```python
from build123d import *

# Parameters (mm, degrees)
F0_R     = 1.27
F1_DEPTH = 1.5875
F0_W     = 8.382
F0_H     = 7.62
F0_W_2   = 0.762
F2_DEPTH = 6.35
F0_W_3   = 11.811
F0_H_2   = 9.017
F0_W_4   = 3.048
F3_DEPTH = 9.525


with BuildPart() as f1:
    # F0 (on Top) → F1 (new body)
    with BuildSketch(Plane.XY):
        Polygon((-34.29, -26.67), (31.79811, -26.67), (31.79811, -25.4), (34.314021, -22.884089), (34.314021, 11.430663), (31.774021, 13.970663), (31.774021, 24.13), (29.21, 26.67), (-34.29, 26.67), (-34.29, 16.002), (-25.908, 16.002), (-25.908, 8.382), (-34.29, 8.382), (-34.29, -13.462), (-22.479, -13.462), (-22.479, -22.479), (-34.29, -22.479), align=None)
        with Locations((-20.32, -24.13)):
            Circle(F0_R, mode=Mode.SUBTRACT)
        with Locations((31.75, -19.05)):
            Circle(F0_R, mode=Mode.SUBTRACT)
        with Locations((-19.05, 24.13)):
            Circle(F0_R, mode=Mode.SUBTRACT)
        with Locations((31.75, 8.89)):
            Circle(F0_R, mode=Mode.SUBTRACT)
    extrude(amount=F1_DEPTH)

    # F0 (on Top) → F2 (join)
    with BuildSketch(Plane.XY):
        with Locations((-30.099, 12.192)):
            Rectangle(F0_W, F0_H)
        with Locations((-34.671, 12.192)):
            Rectangle(F0_W_2, F0_H)
    extrude(amount=F2_DEPTH)

    # F0 (on Top) → F3 (join)
    with BuildSketch(Plane.XY):
        with Locations((-28.3845, -17.9705)):
            Rectangle(F0_W_3, F0_H_2)
        with Locations((-35.814, -17.9705)):
            Rectangle(F0_W_4, F0_H_2)
    extrude(amount=F3_DEPTH)


solid = f1.part
```
Part model, mm, in its own coordinate system. A direction names the side the tool comes from. Give positions to 0.01 mm unless a question says otherwise; leave off trailing zeros. Write each loop counter-clockwise with the first axis right and the second up, starting at its lowest first coordinate (ties: lowest second). Pieces come first, ordered by that corner, then holes. Notation, with made-up numbers: M 23,-20.5 L 27,-20.5 A8 ccw 27,-9.5 Z; hole C 15,71.5 d2. An arc over 180 degrees is marked long. Use CSV: the item, a comma, the result in double quotes.
Item 1: Drill centre lines: probe 1 along Z at (x, y) = (-3, -6); probe 2 along X at (y, z) = (-17, 5.5); probe 3 along Y at (x, z) = (-21, 1.25). Where is each one in solid material? Low to high.
Taken from the geometry:
probe 1,"z = 0 to 1.59"
probe 2,"x = -37.34 to -22.48"
probe 3,"y = -26.67 to -25.2, -23.06 to 26.67"
Item 2: Slice it at D-D on z = 7.5. Write the cut outline in (x, y).
Taken from the geometry:
outline,"M -37.34,-22.48 L -22.48,-22.48 L -22.48,-13.46 L -37.34,-13.46 Z"
Item 3: Slice it at C-C on x = -25. Write the cut outline in (y, z) (1 decimal), plus the area to 3 significant figures.
Taken from the geometry:
outline,"M -26.7,0 L 26.7,0 L 26.7,1.6 L -13.5,1.6 L -13.5,9.5 L -22.5,9.5 L -22.5,1.6 L -26.7,1.6 Z"
area,"156 mm²"
Item 4: Slice it at B-B on z = 2.75. Write the cut outline in (x, y).
Taken from the geometry:
outline,"M -37.34,-22.48 L -22.48,-22.48 L -22.48,-13.46 L -37.34,-13.46 Z; M -35.05,8.38 L -25.91,8.38 L -25.91,16 L -35.05,16 Z"
Item 5: Which spindle directions (+Z, -Z, +X, -X, +Y, -Y) get a long thin tool onto all of the face, cutting with end or side? Do faces 5 (the face through (-31, 12, 6.35)), 6 (the face through (-34.29, -25, 1)), 7 (the face through (31.774, 19, 1)), 8 (the face through (-35.052, 12, 3)). Say none if no direction does.
Taken from the geometry:
face 5,"+Z, +X, -X, +Y"
face 6,"+Z, -Z, -X, -Y"
face 7,"+Z, -Z, +X, +Y"
face 8,"+Z, -Z, -X, +Y"
Item 6: Slice it at A-A on y = -19.05. Write the cut outline in (x, z) (1 decimal).
Taken from the geometry:
outline,"M -37.3,0 L 30.5,0 L 30.5,1.6 L -22.5,1.6 L -22.5,9.5 L -37.3,9.5 Z; M 33,0 L 34.3,0 L 34.3,1.6 L 33,1.6 Z"
Item 7: Pin check, flat tips, straight feed: P1, Ø1.3, axis at y = 18, z = 0.5, coming from the +X side; P2, Ø1.9, axis at y = 12.5, z = 2, coming from the -X side; P3, Ø2.5, axis at x = -31, y = 13, coming from the +Z side. Stop position of each tip, or through.
Taken from the geometry:
P1,"stops at x = 31.77"
P2,"stops at x = -35.05"
P3,"stops at z = 6.35"
Item 8: Pull direction X, two halves, no side cores. Call faces 1 (the face through (-37.338, -18, 5)), 2 (the face through (33, -24.2, 0.8)), 3 (the face through (-30, -22.479, 6)), 4 (the face through (-21.256, -23.272, 0.783)): +X half, -X half, draft (parallel to the pull), parting line (faces both ways), or undercut.
Taken from the geometry:
face 1,"-X half"
face 2,"+X half"
face 3,"draft"
face 4,"undercut"
